Drawing for the job (mm, zero at the part's lowest x, y, z). A direction names the side the tool comes from. Coordinates: 2 decimals unless noted, no trailing zeros. Loops run counter-clockwise (first coordinate to the right, second up) from the corner with the lowest first, then second, coordinate; pieces in that order, holes last. Notation, with made-up numbers: (82.25, -16.5) - (116.25, -16.5) arc R5 cw to (116.25, -8.5) - close; hole circle Ø8 at (18, 50.5). An arc over 180 degrees is marked (long way). Put each result on its own line as item: value.
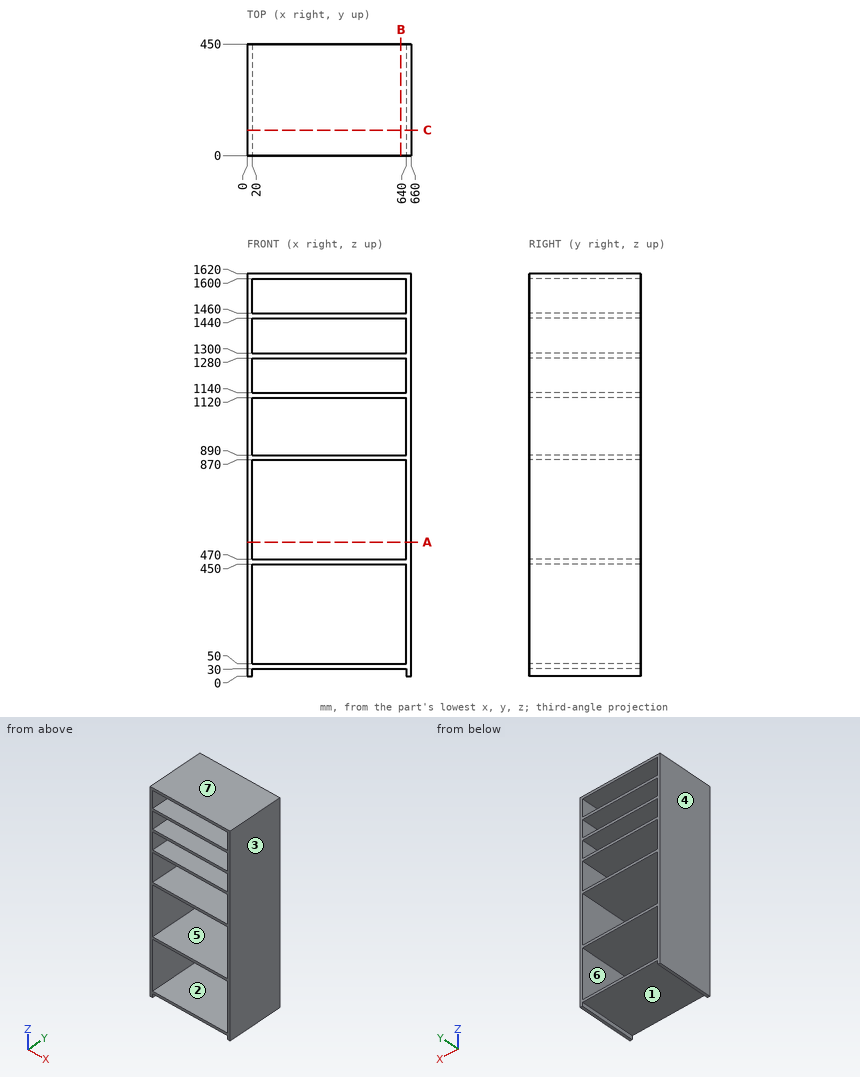
Q1. Wall check: L1, parallel to X at y = 254.5, z = 953. Give the ranges that are in metal, low to high. Write a range as from..to.
Determined:
L1: 0..20, 640..660
Q2. Slice it at C-C, the plane y = 103. State how many separate pieces and enclosed holes the cut face has, then the cut area to 3 significant figures.
Determined:
separate pieces: 1
enclosed holes: 6
area: 152,000 mm2
Q3. Slice it at B-B, the plane x = 619. Give the cut face in (y, z), then the cut area to 3 significant figures.
Determined:
outline: (0, 30) - (450, 30) - (450, 50) - (0, 50) - close; (0, 450) - (450, 450) - (450, 470) - (0, 470) - close; (0, 870) - (450, 870) - (450, 890) - (0, 890) - close; (0, 1120) - (450, 1120) - (450, 1140) - (0, 1140) - close; (0, 1280) - (450, 1280) - (450, 1300) - (0, 1300) - close; (0, 1440) - (450, 1440) - (450, 1460) - (0, 1460) - close; (0, 1600) - (450, 1600) - (450, 1620) - (0, 1620) - close
area: 63,000 mm2
Q4. Tool access for the marked faces 1, 2 and 3: list every direction of +Z, -Z, +X, -X, +Y, -Y with a clear straight run to the whole face (end or side of a thin tool).
Determined:
face 1: -Z, +Y, -Y
face 2: +Y, -Y
face 3: +Z, -Z, +X, +Y, -Y
Q5. Pin check, flat tip, straight feed: pin 1 Ø1.5 at (x, y) = (296.5, 108) entering from -Z. Stop position of the tip, or through.
Determined:
pin 1: z = 30
Q6. Mould opens along X. For the marked faces 4, 5, 6 and 7 say: +X half, -X half, draft (parallel to the pull), parting line (faces both ways), or undercut.
Determined:
face 4: -X half
face 5: undercut
face 6: undercut
face 7: draft
Q7. Slice it at A-A, the plane z = 539.5. Give the cut face in (x, y).
Determined:
outline: (0, 0) - (20, 0) - (20, 450) - (0, 450) - close; (640, 0) - (660, 0) - (660, 450) - (640, 450) - close
